Verification items for the finished model (mm, model axes). Face numbers are marked on the shaded views. A direction names the side the tool comes from. Coordinates: 2 decimals unless noted, no trailing zeros. Loops run counter-clockwise (first coordinate to the right, second up) from the corner with the lowest first, then second, coordinate; pieces in that order, holes last.
Q1. Sectioned sample at A-A (z = 5.2). Enter the section's corners in (x, y), then the cut area to 3 significant figures.
Q2. Access from +Z, -Z, +X, -X, +Y, -Y to the whole of each face (thin tool, end or side, straight path). Record for the marked faces 1, 2 and 3.
Q3. Material ranges on probe 1 along Z at (x, y) = (-8, -6); probe 2 along X at (y, z) = (-3, 4.95); probe 3 along X at (y, z) = (3.25, 1.95), recorded low to high.
Q4. Go/stop test with flat-tipped pins: P1, Ø4, axis at x = 5.5, y = -5, coming from the -Z side; P2, Ø10, axis at x = -3, y = -2, coming from the -Z side; P3, Ø5, axis at x = 5.5, y = 4.5, coming from the +Z side. Record where each tip stops, or that it passes through.
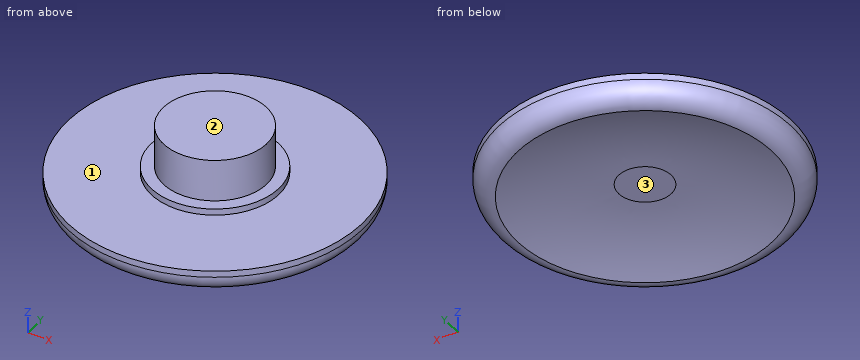
```python
from build123d import *

# Parameters (mm, degrees)
F0_R     = 11.5
F1_DEPTH = 2
F2_R     = 5
F3_DEPTH = 0.5
F4_R     = 4.05
F5_DEPTH = 3.3
F6_R     = 10
F7_DEPTH = 1
F9_R     = 1.49999


# Not quite as in the source:
# - a fillet or chamfer that OpenCascade refuses, or shapes differently, is made with other operations: its cross-section is extruded or revolved along the edge and cut away or added
# - a fillet or chamfer is up to 0.001 mm smaller than in the source, because OpenCascade refuses the exact size


with BuildPart() as f1:
    # F0 (on Top) → F1 (new body)
    with BuildSketch(Plane.XY):
        Circle(F0_R)
    extrude(amount=F1_DEPTH)

    # F2 (on face) → F3 (join)
    with BuildSketch(Plane.XY.offset(2)):
        Circle(F2_R)
    extrude(amount=F3_DEPTH)

    # F4 (on face) → F5 (join)
    with BuildSketch(Plane.XY.offset(2.5)):
        Circle(F4_R)
    extrude(amount=F5_DEPTH)

    # F6 (on face) → F7 (cut)
    with BuildSketch(Plane(origin=(0, 0, 0), x_dir=(1, 0, 0), z_dir=(0, 0, -1))):
        Circle(F6_R)
    extrude(amount=-F7_DEPTH, mode=Mode.SUBTRACT)

    # F8: fillet of radius 32 on 1 edges, made by hand

    # F8_s1 → F8_t2 (revolve)
    with BuildSketch(Plane.XZ):
        with BuildLine():
            ThreePointArc((10, 0), (6.0627460668, 0.7490157328), (2.0627460668, 1))
            Line((2.0627460668, 1), (10, 1))
            Line((10, 1), (10, 0))
        make_face()
    revolve(axis=Axis((0, 0, 1), (0, 0, -1)))

    # F9 (radius 1.5 in the source; OpenCascade refuses exactly that, so slightly less here)
    f9_edges = [f1.edges().sort_by_distance(p)[0] for p in [
        (-11.5, 0, 0),
    ]]
    fillet(f9_edges, radius=F9_R)


solid = f1.part
```
Geometry check:
1. outline: circle Ø8.1 at (0, 0)
1. area: 51.5 mm2
2. face 1: +Z
2. face 2: +Z, +X, -X, +Y, -Y
2. face 3: -Z
3. probe 1: z = 0 to 2
3. probe 2: x = -2.72 to 2.72
3. probe 3: x = -11.03 to 11.03
4. P1: stops at z = 0.14
4. P2: stops at z = 0.32
4. P3: stops at z = 2.5
